```python
from build123d import *

# Parameters (mm, degrees)
EXTRU_MINCE1_DEPTH        = 100
CONVERTIR_VOLUME1_DEPTH   = 100
CONVERTIR_VOLUME1_2_DEPTH = 100


# Read off the part's stored shape, not the designer's step: Convertir-Volume1
with BuildPart() as part:
    # Esquisse1 → Extru.-Mince1 (new body)
    with BuildSketch(Plane.XY):
        Polygon((-133.505441468, 147.472825463), (-133.505441468, 87.472825463), (-233.505441468, 87.472825463), (-233.505441468, -82.527174537), (-133.505441468, -82.527174537), (-133.505441468, -142.527174537), (-123.505441468, -142.527174537), (-123.505441468, -72.527174537), (-223.505441468, -72.527174537), (-223.505441468, 77.472825463), (-123.505441468, 77.472825463), (-123.505441468, 147.472825463), align=None)
    extrude(amount=EXTRU_MINCE1_DEPTH)

    # Convertir-Volume1 outline → Convertir-Volume1 (cut)
    with BuildSketch(Plane.XY):
        with BuildLine():
            Line((-123.505441468, 147.472825463), (-133.505441468, 147.472825463))
            Line((-133.505441468, 147.472825463), (-133.505441468, 87.472825463))
            Line((-133.505441468, 87.472825463), (-232.505441468, 87.472825463))
            ThreePointArc((-232.505441468, 87.472825463), (-233.212548249, 87.179932244), (-233.505441468, 86.472825463))
            Line((-233.505441468, 86.472825463), (-233.505441468, -81.527174537))
            ThreePointArc((-233.505441468, -81.527174537), (-233.212548249, -82.234281318), (-232.505441468, -82.527174537))
            Line((-232.505441468, -82.527174537), (-133.505441468, -82.527174537))
            Line((-133.505441468, -82.527174537), (-133.505441468, -142.527174537))
            Line((-133.505441468, -142.527174537), (-123.505441468, -142.527174537))
            Line((-123.505441468, -142.527174537), (-123.505441468, -72.527174537))
            Line((-123.505441468, -72.527174537), (-223.505441468, -72.527174537))
            Line((-223.505441468, -72.527174537), (-223.505441468, 77.472825463))
            Line((-223.505441468, 77.472825463), (-123.505441468, 77.472825463))
            Line((-123.505441468, 77.472825463), (-123.505441468, 147.472825463))
        make_face()
    extrude(amount=CONVERTIR_VOLUME1_DEPTH, mode=Mode.SUBTRACT)

    # Convertir-Volume1 2 outline → Convertir-Volume1 2 (add)
    with BuildSketch(Plane.XY):
        with BuildLine():
            Line((-133.505441468, 147.472825463), (-135.505441468, 147.472825463))
            Line((-135.505441468, 147.472825463), (-135.505441468, 90.472825463))
            ThreePointArc((-135.505441468, 90.472825463), (-135.798334686, 89.765718682), (-136.505441468, 89.472825463))
            Line((-136.505441468, 89.472825463), (-232.505441468, 89.472825463))
            ThreePointArc((-232.505441468, 89.472825463), (-234.626761811, 88.594145807), (-235.505441468, 86.472825463))
            Line((-235.505441468, 86.472825463), (-235.505441468, -81.527174537))
            ThreePointArc((-235.505441468, -81.527174537), (-234.626761811, -83.64849488), (-232.505441468, -84.527174537))
            Line((-232.505441468, -84.527174537), (-136.505441468, -84.527174537))
            ThreePointArc((-136.505441468, -84.527174537), (-135.798334686, -84.820067756), (-135.505441468, -85.527174537))
            Line((-135.505441468, -85.527174537), (-135.505441468, -142.527174537))
            Line((-135.505441468, -142.527174537), (-133.505441468, -142.527174537))
            Line((-133.505441468, -142.527174537), (-133.505441468, -85.527174537))
            ThreePointArc((-133.505441468, -85.527174537), (-134.384121124, -83.405854193), (-136.505441468, -82.527174537))
            Line((-136.505441468, -82.527174537), (-233.505441468, -82.527174537))
            Line((-233.505441468, -82.527174537), (-233.505441468, 87.472825463))
            Line((-233.505441468, 87.472825463), (-136.505441468, 87.472825463))
            ThreePointArc((-136.505441468, 87.472825463), (-134.384121124, 88.351505119), (-133.505441468, 90.472825463))
            Line((-133.505441468, 90.472825463), (-133.505441468, 147.472825463))
        make_face()
    extrude(amount=CONVERTIR_VOLUME1_2_DEPTH)


solid = part.part
```
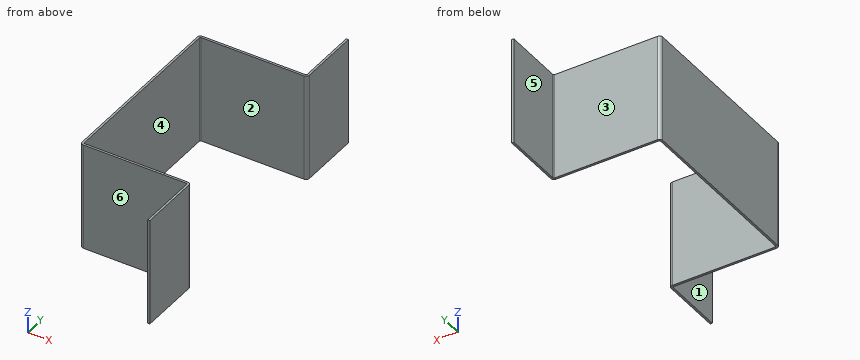
Here's how the part is built. I have some questions about the finished solid (model axes, mm). Face numbers are marked on the shaded views. A direction names the side the tool comes from. Round coordinates to 2 decimals unless told otherwise and drop trailing zeros. Order: outer loops, then holes, each group sorted by start corner. A loop starts at its lowest first (then second) coordinate and runs counter-clockwise, first axis right, second up. Notation, with made-up numbers: (4.25, 52) -> (27.25, 52) arc R29 ccw to (27.25, 74) -> close; hole circle Ø9 at (23.5, 64.25). An arc over 180 degrees is marked (long way). Use a Markdown table: item, result. Add a question column.
(1) Suppose I cut it at C-C, the plane y = -117. Please give me the cut outline in (x, z), and give its area (3 significant figures).
(2) Suppose I cut it at B-B, the plane z = 20.5. Please give me the cut outline in (x, y), and give its area (3 significant figures).
(3) I need wall thicknesses on line 1 along Y through (x, z) = (-155, 26); line 2 along X through (y, z) = (-36.5, 16); line 3 along X through (y, z) = (132.5, 79). Which ranges of each line are inside material? Lowest first, please.
(4) For pin 1 Ø10 at (x, z) = (-178.5, 81.5) entering from +Y; pin 2 Ø17 at (y, z) = (119, 39.5) entering from -X; pin 3 Ø1.5 at (x, z) = (-201.5, 27.5) entering from -Y; pin 4 Ø8 at (x, y) = (-154, 94.5) entering from -Z, each with a flat end and sliding along its axis, tell me the tip position at first contact or that it passes through.
(5) If we mould it in two halves opening along Y, with no side actions, what happens to the marked faces 4, 5 and 6? For each: released by +Y, released by -Y, zero draft, split by the parting line, or undercut.
(6) Suppose I cut it at A-A, the plane x = -211. Please give me the cut outline in (y, z), and give its area (3 significant figures).
(7) For the marked faces 1, 2 and 3, which set-ups out of +Z, -Z, +X, -X, +Y, -Y let a thin tool reach every point of the face, with its end or its side?
Verdict:
| question | item | result |
|---|---|---|
| 1 | outline | (-135.51, 0) -> (-133.51, 0) -> (-133.51, 100) -> (-135.51, 100) -> close |
| 1 | area | 200 mm2 |
| 2 | outline | (-235.51, -81.53) arc R3 ccw to (-232.51, -84.53) -> (-136.51, -84.53) arc R1 cw to (-135.51, -85.53) -> (-135.51, -142.53) -> (-133.51, -142.53) -> (-133.51, -85.53) arc R3 ccw to (-136.51, -82.53) -> (-232.51, -82.53) arc R1 cw to (-233.51, -81.53) -> (-233.51, 86.47) arc R1 cw to (-232.51, 87.47) -> (-136.51, 87.47) arc R3 ccw to (-133.51, 90.47) -> (-133.51, 147.47) -> (-135.51, 147.47) -> (-135.51, 90.47) arc R1 cw to (-136.51, 89.47) -> (-232.51, 89.47) arc R3 ccw to (-235.51, 86.47) -> close |
| 2 | area | 973 mm2 |
| 3 | line 1 | -84.53 to -82.53, 87.47 to 89.47 |
| 3 | line 2 | -235.51 to -233.51 |
| 3 | line 3 | -135.51 to -133.51 |
| 4 | pin 1 | y = 89.47 |
| 4 | pin 2 | x = -135.51 |
| 4 | pin 3 | y = -84.53 |
| 4 | pin 4 | through |
| 5 | face 4 | undercut |
| 5 | face 5 | zero draft |
| 5 | face 6 | released by -Y |
| 6 | outline | (-84.53, 0) -> (-82.53, 0) -> (-82.53, 100) -> (-84.53, 100) -> close; (87.47, 0) -> (89.47, 0) -> (89.47, 100) -> (87.47, 100) -> close |
| 6 | area | 400 mm2 |
| 7 | face 1 | +Z, -Z, -X, -Y |
| 7 | face 2 | +Z, -Z, +X |
| 7 | face 3 | +Z, -Z, -X, +Y |
